Autodesk Inventor part; units mm, degrees
ref_plane "Work Plane1" through (0, 0, -15) normal (0, 0, 1) x (1, 0, 0)
ref_plane "YZ Plane" through (0, 0, 0) normal (1, 0, 0) x (0, 1, 0)
ref_plane "XZ Plane" through (0, 0, 0) normal (0, 1, 0) x (-1, 0, 0)
sketch "Sketch1" plane through (0, 0, 0) normal (0, 0, 1) x (1, 0, 0)
  line L0 (0, 0) -> (25, 0)
  line L1 (25, 0) -> (25, 40)
  line L2 (25, 40) -> (0, 40)
  line L3 (0, 40) -> (0, 0)
  dimension "d1" = 25
  dimension "d2" = 40
  dimension "d3" = 25
extrude "Extrusion1" add sketch "Sketch1" against normal blind 30
sketch "Sketch2" plane through (25, 0, 0) normal (1, 0, 0) x (0, 0, -1)
  line L0 (0, 0) -> (30, 0)
  circle A0 centre (15, 6.56) radius 2.46
extrude "Extrusion2" cut sketch "Sketch2" against normal blind 30
sketch "Sketch3" plane through (0, 0, 0) normal (-1, 0, 0) x (0, 0, 1)
  line L0 (0, 0) -> (-30, 0)
  line L1 (-25.05, 0) -> (-4.95, 0)
  line L2 (-4.95, 0) -> (-4.95, 33.12)
  line L3 (-4.95, 33.12) -> (-25.05, 33.12)
  line L4 (-25.05, 33.12) -> (-25.05, 0)
  dimension "d11" = 20.1
extrude "Extrusion3" cut sketch "Sketch3" against normal blind 20
sketch "Sketch4" plane through (0, 0, 0) normal (0, -1, 0) x (1, 0, 0)
  line L0 (20, -4.95) -> (20, -25.05)
  line L1 (20, -15) -> (25, -15)
  line L2 (25, 0) -> (25, -30)
  line L3 (20, -8.025) -> (25, -8.025)
  line L4 (25, -8.025) -> (25, -21.975)
  line L5 (25, -21.975) -> (20, -21.975)
  line L6 (20, -21.975) -> (20, -8.025)
  line L7 (20, -8.025) -> (25, -21.975) construction
  line L8 (25, -8.025) -> (20, -21.975) construction
  line L9 (25, -12.54) -> (25, -17.46)
  point P0 (0, 0)
  point P1 (22.5, -15)
  dimension "d14" = 13.95
extrude "Extrusion4" add sketch "Sketch4" along normal blind 15
sketch "Sketch5" plane through (20, 0, 0) normal (-1, 0, 0) x (0, 0, 1)
  circle A0 centre (-15, 6.56) radius 2.46
  circle A1 centre (-15, 6.56) radius 4.7025
  circle A2 centre (-15, 6.56) radius 2.46
  circle A3 centre (-15, 6.56) radius 2.46
  point P0 (0, 0)
  dimension "d17" = 9.405
extrude "Extrusion5" cut sketch "Sketch5" against normal blind 2.1
sketch "Sketch6" plane through (25, 0, 0) normal (1, 0, 0) x (0, 0, -1)
  circle A0 centre (15, 6.56) radius 4.7025
  line L0 (15, 6.56) -> (15, 23.56)
  circle A1 centre (15, 23.56) radius 2.46
  point P0 (0, 0)
  dimension "d20" = 17
  dimension "d21" = 4.92
extrude "Extrusion6" cut sketch "Sketch6" against normal blind 10 contours A1
sketch "Sketch7" plane through (20, 0, 0) normal (-1, 0, 0) x (0, 0, 1)
  circle A0 centre (-15, 23.56) radius 2.46
  circle A1 centre (-15, 23.56) radius 4.7025
  point P0 (0, 0)
  dimension "d24" = 9.405
extrude "Extrusion7" cut sketch "Sketch7" against normal blind 2.1
sketch "Sketch9" plane through (25, 0, 0) normal (1, 0, 0) x (0, 0, -1)
  circle A0 centre (15, 6.56) radius 2.46
  circle A1 centre (15, 6.56) radius 2.46
  circle A2 centre (15, 23.56) radius 2.46
  circle A3 centre (15, 23.56) radius 2.46
  line L0 (30, 40) -> (30, 0)
  line L1 (30, 0) -> (30, 40)
  line L2 (30, 40) -> (0, 40)
  line L3 (0, 40) -> (0, 0)
  line L4 (0, 0) -> (8.025, 0)
  line L5 (21.975, 0) -> (21.975, -15)
  line L6 (21.975, -15) -> (8.025, -15)
  line L7 (8.025, -15) -> (8.025, 0)
  line L8 (0, 0) -> (8.025, 0)
  line L9 (21.975, 0) -> (30, 0)
extrude "Extrusion8" add sketch "Sketch9" along normal blind 5
sketch "Sketch10" plane through (0, 40, 0) normal (0, 1, 0) x (1, 0, 0)
  line L0 (0, 30) -> (30, 30)
  line L1 (30, 0) -> (0, 0)
  line L2 (0, 30) -> (30, 30)
  line L3 (30, 30) -> (30, 0)
  line L4 (30, 0) -> (0, 0)
  line L5 (0, 0) -> (0, 30)
extrude "Extrusion9" add sketch "Sketch10" along normal blind 30
sketch "Sketch12" plane through (30, 0, 0) normal (1, 0, 0) x (0, 0, -1)
  circle A0 centre (15, 6.56) radius 2.46
  line L0 (15, 6.56) -> (15, 15.06)
  circle A1 centre (15, 15.06) radius 2.525
  point P0 (0, 0)
  dimension "d31" = 8.5
  dimension "d33" = 5.05
extrude "Extrusion10" cut sketch "Sketch12" against normal blind 30 contours A1
sketch "Sketch15" plane through (0, 0, -25.05) normal (-1, 0, 0) x (0, 0, 1)
  line L0 (0, 33.12) -> (20.1, 33.12)
  line L1 (20.1, 33.12) -> (20.1, 0)
  line L2 (0, 33.12) -> (20.1, 33.12)
  line L3 (20.1, 33.12) -> (20.1, 31.1)
  line L4 (20.1, 31.1) -> (0, 31.1)
  line L5 (0, 31.1) -> (0, 33.12)
  point P0 (25.05, 0)
  dimension "d57" = 2.02
extrude "Extrusion13" add sketch "Sketch15" against normal blind 20
sketch "Sketch17" plane through (0, 0, 0) normal (0, 0, 1) x (1, 0, 0)
  line L0 (0, 70) -> (30, 70)
  line L1 (30, 70) -> (50.0622, 90.0622)
  line L2 (30, 70) -> (80, 70) construction
  line L3 (11.9522, 97.2454) -> (0, 85.2932)
  line L4 (0, 70) -> (0, 85.2932)
  line L5 (0, 70) -> (0, 0)
  line L6 (0, 70) -> (30, 70)
  line L7 (10.923, 112.2849) -> (0, 120.567)
  line L8 (50.0622, 105.3553) -> (50.0622, 120.567)
  line L9 (50.0622, 105.3553) -> (50.0622, 90.0622)
  arc A0 (11.9522, 97.2454) -> (10.923, 112.2849) centre (4.8811, 104.3165) ccw
  line L10 (4, 138.567) -> (0, 140.567)
  line L11 (4, 122.567) -> (0, 120.567)
  line L12 (4, 122.567) -> (8, 130.567)
  line L13 (4, 138.567) -> (8, 130.567)
  line L14 (0, 140.567) -> (30, 140.567)
  line L15 (30, 140.567) -> (50.0622, 120.567)
  dimension "d61" = 45
  dimension "d62" = 32.0271
  dimension "d72" = 10
extrude "Extrusion14" add sketch "Sketch17" against normal blind 30
sketch "Sketch21" plane through (0, 0, 0) normal (0, 0, 1) x (1, 0, 0)
  line L0 (50.0622, 90.0622) -> (30, 70)
  line L1 (30, 70) -> (50.0622, 90.0622)
  line L2 (50.0622, 90.0622) -> (50.0622, 120.567)
  line L3 (50.0622, 90.0622) -> (50.0622, 120.567)
  line L4 (0, 140.567) -> (30, 140.567)
  line L5 (50.0622, 120.567) -> (30, 140.567)
  line L6 (30, 140.567) -> (0, 140.567)
  line L7 (4, 138.567) -> (0, 140.567)
  line L8 (0, 140.567) -> (4, 138.567)
  line L9 (8, 130.567) -> (4, 138.567)
  line L10 (4, 138.567) -> (8, 130.567)
  line L11 (4, 122.567) -> (8, 130.567)
  line L12 (8, 130.567) -> (4, 122.567)
  line L13 (0, 120.567) -> (4, 122.567)
  line L14 (4, 122.567) -> (0, 120.567)
  line L15 (10.923, 112.2849) -> (0, 120.567)
  line L16 (0, 120.567) -> (10.923, 112.2849)
  line L17 (0, 85.2932) -> (11.9522, 97.2454)
  line L18 (11.9522, 97.2454) -> (0, 85.2932)
  line L19 (0, 85.2932) -> (0, 55.2932)
  line L20 (0, 55.2932) -> (30, 55.2932)
  line L21 (30, 55.2932) -> (30, 70)
  arc A0 (11.9522, 97.2454) -> (10.923, 112.2849) centre (4.8811, 104.3165) ccw
  dimension "d79" = 30
  dimension "d81" = 30
extrude "Extrusion15" add sketch "Sketch21" along normal blind 45
ref_plane "Work Plane1" through (0, 0, -15) normal (0, 0, 1) x (1, 0, 0)
mirror "Mirror1" about plane through (0, 0, -15) normal (0, 0, 1) of "Extrusion15"
properties part number "rec_c_16mm_x_120mm"
The listing builds one solid part. Answer for the finished solid, in the listing's coordinates (mm). A direction names the side the tool comes from. Give positions to 0.01 mm unless a question says otherwise; leave off trailing zeros. Write each loop counter-clockwise with the first axis right and the second up, starting at its lowest first coordinate (ties: lowest second). Pieces come first, ordered by that corner, then holes.
1) A tool of negligible diameter and unlimited length cuts with its end or side. For faces 1 (the face through (2.03, 121.58, -14.16)), 2 (the face through (15, 28, 0)), 3 (the face through (25, -7, -21.975)), 4 (the face through (10, 31.1, -15)), from which of +Z, -Z, +X, -X, +Y, -Y can it reach the whole face along a straight path? Write none if from no direction.
2) Section D-D (z = -55) is taken. Write down the section's boundary in (x, y), and give its area (3 significant figures).
3) Find the intervals of material crossed by L1, parallel to Y at x = 27.5, z = -15 (3 decimals); L2, parallel to Y at x = 21.75, z = -15 (1 decimal); L3, parallel to Z at x = 4, y = 5.5, in increasing order.
4) Section B-B (x = 6) is taken. Write down the section's boundary in (y, z).
5) Section A-A (y = 23.56) is taken. Write down the section's boundary in (x, z), and give its area (3 significant figures).
6) Given P1, Ø5, axis at x = 25, y = -11, coming from the -Z side (3 decimals); P2, Ø10, axis at x = 12.5, y = 23, coming from the +Z side; P3, Ø6, axis at y = 115.5, z = -39, coming from the -X side, each flat-ended and moving along its own axis, determine where each tip first touches the part or whether it passes through.
7) Section C-C (x = 26.5) is taken. Write down the section's boundary in (y, z) (3 decimals).
8) For a pull along Z with two mould halves and no side action, classify faces 5 (the face through (25.995, 7.502, -17.272)), 6 (the face through (15, 28, -30)), 7 (the face through (5.972, 134.623, -14.16)) as pulls with the +Z half, pulls with the -Z half, needs draft (parallel to the pull), parting line crosses it, or undercut.
Response:
1. face 1: +Z, -Z, -X
1. face 2: +Z, +X, -X, -Y
1. face 3: -Z, +X, -X, -Y
1. face 4: -X, -Y
2. outline: (0, 55.29) - (30, 55.29) - (30, 70) - (50.06, 90.06) - (50.06, 120.57) - (30, 140.57) - (0, 140.57) - (4, 138.57) - (8, 130.57) - (4, 122.57) - (0, 120.57) - (10.92, 112.28) arc R10 cw to (11.95, 97.25) - (0, 85.29) - close
2. area: 3,140 mm2
3. L1: y = -15 to 4.1, 9.02 to 12.535, 17.585 to 21.1, 26.02 to 140.567
3. L2: y = -15 to 1.9, 11.3 to 12.5, 17.6 to 18.9, 28.3 to 140.6
3. L3: z = -30 to -25.05, -4.95 to 0
4. outline: (0, -30) - (55.29, -30) - (55.29, -75) - (91.29, -75) - (91.29, 45) - (55.29, 45) - (55.29, 0) - (0, 0) - (0, -4.95) - (31.1, -4.95) - (31.1, -25.05) - (0, -25.05) - close; (116.02, -75) - (126.57, -75) - (126.57, 45) - (116.02, 45) - close; (134.57, -75) - (140.57, -75) - (140.57, 45) - (134.57, 45) - close
5. outline: (0, -30) - (30, -30) - (30, -17.46) - (22.1, -17.46) - (22.1, -19.7) - (20, -19.7) - (20, -25.05) - (0, -25.05) - close; (0, -4.95) - (20, -4.95) - (20, -10.3) - (22.1, -10.3) - (22.1, -12.54) - (30, -12.54) - (30, 0) - (0, 0) - close
5. area: 439 mm2
6. P1: stops at z = -21.975
6. P2: stops at z = 0
6. P3: stops at x = 2.73
7. outline: (-15, -21.975) - (0, -21.975) - (0, -30) - (55.293, -30) - (55.293, -75) - (140.567, -75) - (140.567, 45) - (55.293, 45) - (55.293, 0) - (0, 0) - (0, -8.025) - (-15, -8.025) - close; hole circle Ø4.92 at (6.56, -15); hole circle Ø5.05 at (15.06, -15); hole circle Ø4.92 at (23.56, -15)
8. face 5: undercut
8. face 6: pulls with the -Z half
8. face 7: needs draft
